Could you check a few things on this model? Use its own coordinates, in mm. A direction names the side the tool comes from. Round coordinates to 2 decimals unless told otherwise and drop trailing zeros. Write each loop counter-clockwise with the first axis right and the second up, starting at its lowest first coordinate (ties: lowest second). Pieces come first, ordered by that corner, then holes. Notation, with made-up numbers: M -11.5,58 L 40.5,58 A15 cw 40.5,71 Z; hole C -16,65 d1. An arc over 180 degrees is marked long. One line per item, written item: value. Start each with the question number.
(1) I want a section at C-C on z = 4.25. Please give me the cut outline in (x, y), and give its area (3 significant figures).
(2) Which directions (+Z, -Z, +X, -X, +Y, -Y) give clear straight access to the entire face, cutting with the end or side of a thin tool? Please do faces 1 (the face through (-4, 17.16, 10)), 2 (the face through (-3, 13, 10)), 3 (the face through (5, 13, 10)).
(3) I want a section at B-B on y = 4. Please give me the cut outline in (x, z).
(4) If I drill on L1, parallel to Z at x = 0, y = -10.2; L2, parallel to X at y = -11.25, z = 15; L3, parallel to Y at x = 4.25, z = 4.25, over which ranges is the centre line in solid material (lowest first)?
(5) I want a section at A-A on x = 0. Please give me the cut outline in (y, z).
(6) I want a section at D-D on x = -6. Please give me the cut outline in (y, z).
(7) I'm going to push flat-ended pins straight in: pin 1 Ø7 at (y, z) = (13.2, 4.25) entering from -X; pin 2 Ø5 at (y, z) = (12.5, 16.5) entering from +X; pin 3 Ø4 at (y, z) = (13.2, 15.75) entering from -X (1 decimal); pin 4 Ø4.5 at (y, z) = (11, 11.5) entering from +X. Where does each tip first touch, or does it pass through?
(8) Thinking about a two-plate mould opening in Z: for faces 4 (the face through (-0.8, -9.5, 20)), 5 (the face through (-5, 13, 10)), 6 (the face through (-0.8, -9.5, 0)), 7 (the face through (-3, -11, 5)), which applies, released by +Z, released by -Z, zero draft, split by the parting line, or undercut?
```python
from build123d import *

# Parameters (mm, degrees)
BOSS_EXTRUDE1_DEPTH = 20
SKETCH3_R           = 2.25
CUT_EXTRUDE1_DEPTH  = 16.5
SKETCH5_R           = 2.125
CUT_EXTRUDE2_DEPTH  = 31.659519334
CUT_EXTRUDE6_START  = -6
SKETCH6_R           = 3
CUT_EXTRUDE6_DEPTH  = 44.5


with BuildPart() as part:
    # Sketch1 → Boss-Extrude1 (new body)
    with BuildSketch(Plane.XY):
        with BuildLine():
            Line((-3, 8.485281374), (-3, 17.159519334))
            Line((-3, 17.159519334), (-5, 17.159519334))
            Line((-5, 17.159519334), (-5, 9.233092656))
            ThreePointArc((-5, 9.233092656), (-9.020809276, 5.373546315), (-10.5, 0))
            Line((-10.5, 0), (-10.5, -13.5))
            Line((-10.5, -13.5), (10.5, -13.5))
            Line((10.5, -13.5), (10.5, 0))
            ThreePointArc((10.5, 0), (9.020809276, 5.373546315), (5, 9.233092656))
            Line((5, 9.233092656), (5, 17.159519334))
            Line((5, 17.159519334), (3, 17.159519334))
            Line((3, 17.159519334), (3, 8.485281374))
            ThreePointArc((3, 8.485281374), (0, -9), (-3, 8.485281374))
        make_face()
    extrude(amount=BOSS_EXTRUDE1_DEPTH)

    # Sketch3 → Cut-Extrude1 (cut, through all)
    with BuildSketch(Plane(origin=(5, 0, 0), x_dir=(0, 0, -1), z_dir=(1, 0, 0))):
        with Locations((-15.75, 13.196305995)):
            Circle(SKETCH3_R)
        with Locations((-4.25, 13.196305995)):
            Circle(SKETCH3_R)
    extrude(amount=-CUT_EXTRUDE1_DEPTH, mode=Mode.SUBTRACT)

    # Sketch5 → Cut-Extrude2 (cut, through all)
    with BuildSketch(Plane.XZ.offset(13.5)):
        with Locations((0, 5)):
            Circle(SKETCH5_R)
        with Locations((0, 15)):
            Circle(SKETCH5_R)
    extrude(amount=-CUT_EXTRUDE2_DEPTH, mode=Mode.SUBTRACT)

    # Sketch6 → Cut-Extrude6 (cut)
    with BuildSketch(Plane.XZ.offset(13.5).offset(CUT_EXTRUDE6_START)):
        with Locations((0, 15)):
            Circle(SKETCH6_R)
        with Locations((0, 5)):
            Circle(SKETCH6_R)
    extrude(amount=CUT_EXTRUDE6_DEPTH, mode=Mode.SUBTRACT)


solid = part.part
```
Found:
1. outline: M -10.5,-13.5 L -2.9,-13.5 L -2.9,-8.52 A9 cw -3,8.49 L -3,10.95 L -5,10.95 L -5,9.23 A10.5 ccw -10.5,0 Z; M -5,15.45 L -3,15.45 L -3,17.16 L -5,17.16 Z; M 2.9,-13.5 L 10.5,-13.5 L 10.5,0 A10.5 ccw 5,9.23 L 5,10.95 L 3,10.95 L 3,8.49 A9 cw 2.9,-8.52 Z; M 3,15.45 L 5,15.45 L 5,17.16 L 3,17.16 Z
1. area: 178 mm²
2. face 1: +Z, -Z, +X, -X, +Y
2. face 2: +Z, -Z, +Y
2. face 3: +Z, -Z, +X, +Y
3. outline: M -9.71,0 L -8.06,0 L -8.06,20 L -9.71,20 Z; M 8.06,0 L 9.71,0 L 9.71,20 L 8.06,20 Z
4. L1: z = 0 to 2, 8 to 12, 18 to 20
4. L2: x = -10.5 to -3, 3 to 10.5
4. L3: y = -13.5 to -7.93, 7.93 to 10.95, 15.45 to 17.16
5. outline: M -13.5,0 L -9,0 L -9,2 L -13.5,2 Z; M -13.5,8 L -9,8 L -9,12 L -13.5,12 Z; M -13.5,18 L -9,18 L -9,20 L -13.5,20 Z
6. outline: M -13.5,0 L -6.71,0 L -6.71,20 L -13.5,20 Z; M 6.71,0 L 8.62,0 L 8.62,20 L 6.71,20 Z
7. pin 1: stops at x = -5
7. pin 2: stops at x = 5
7. pin 3: passes through
7. pin 4: stops at x = 5.8
8. face 4: released by +Z
8. face 5: zero draft
8. face 6: released by -Z
8. face 7: undercut
